Can you work these out from the model? Positions are in its coordinate system, mm. A direction names the side the tool comes from. Give positions to 0.01 mm unless a question says otherwise; leave off trailing zeros. Order: outer loops, then holes, each group sorted by start corner. A loop starts at its lowest first (then second) coordinate and runs counter-clockwise, first axis right, second up. Notation, with made-up numbers: (80.5, 46) - (94.5, 46) arc R22 cw to (94.5, 81) - close; hole circle Ø7 at (-21.5, 47). An arc over 180 degrees is marked (long way). Answer as CSV lines item,"result".
```python
from build123d import *

# Parameters (mm, degrees)
SKETCH1_R           = 200
BOSS_EXTRUDE1_DEPTH = 10
SKETCH2_R           = 6.25
CUT_EXTRUDE1_DEPTH  = 284.019433962
SKETCH4_R           = 2.55
CUT_EXTRUDE2_DEPTH  = 284.019433962
CIRPATTERN1_COUNT   = 8
SKETCH5_R           = 2.05
CUT_EXTRUDE3_DEPTH  = 284.019433962
CIRPATTERN2_COUNT   = 4
CUT_EXTRUDE4_START  = -10
CUT_EXTRUDE4_DEPTH  = 10
CIRPATTERN3_COUNT   = 4
SKETCH7_R           = 40
CUT_EXTRUDE5_DEPTH  = 282.602556807
FILLET1_R           = 10


with BuildPart() as part:
    # Sketch1 → Boss-Extrude1 (new body)
    with BuildSketch(Plane(origin=(0, 0, 0), x_dir=(1, 0, 0), z_dir=(0, 1, 0))):
        with Locations(Location((0, 0, 0), (0, 0, 270))):
            Circle(SKETCH1_R)
    extrude(amount=BOSS_EXTRUDE1_DEPTH)

    # Sketch2 → Cut-Extrude1 (cut, through all)
    with BuildSketch(Plane(origin=(0, 10, 0), x_dir=(1, 0, 0), z_dir=(0, 1, 0))):
        with Locations(Location((-135.764501988, 0, 0), (0, 0, 270))):
            Circle(SKETCH2_R)
        with Locations(Location((0, -135.764501988, 0), (0, 0, 270))):
            Circle(SKETCH2_R)
        with Locations(Location((135.764501988, 0, 0), (0, 0, 270))):
            Circle(SKETCH2_R)
        with Locations(Location((0, 135.764501988, 0), (0, 0, 270))):
            Circle(SKETCH2_R)
    extrude(amount=-CUT_EXTRUDE1_DEPTH, mode=Mode.SUBTRACT)

    # Sketch4 → Cut-Extrude2 (cut, through all)
    with BuildSketch(Plane(origin=(0, 10, 0), x_dir=(1, 0, 0), z_dir=(0, 1, 0))):
        with Locations(Location((20.090880199, 48.503675457, 0), (0, 0, 270))):
            Circle(SKETCH4_R)
    cut_extrude2 = extrude(amount=-CUT_EXTRUDE2_DEPTH, mode=Mode.SUBTRACT)

    # CirPattern1: Cut-Extrude2 ×8 about axis
    cirpattern1_axis = Axis((0, 0, 0), (0, 1, 0))
    for i in range(1, CIRPATTERN1_COUNT):
        add(cut_extrude2.rotate(cirpattern1_axis, i * 360 / CIRPATTERN1_COUNT), mode=Mode.SUBTRACT)

    # Sketch5 → Cut-Extrude3 (cut, through all)
    with BuildSketch(Plane(origin=(0, 10, 0), x_dir=(1, 0, 0), z_dir=(0, 1, 0))):
        with Locations(Location((-188.264501988, 8.25, 0), (0, 0, 270))):
            Circle(SKETCH5_R)
        with Locations(Location((-174.764501988, 8.25, 0), (0, 0, 270))):
            Circle(SKETCH5_R)
        with Locations(Location((-174.764501988, -8.25, 0), (0, 0, 270))):
            Circle(SKETCH5_R)
        with Locations(Location((-188.264501988, -8.25, 0), (0, 0, 270))):
            Circle(SKETCH5_R)
    cut_extrude3 = extrude(amount=-CUT_EXTRUDE3_DEPTH, mode=Mode.SUBTRACT)

    # CirPattern2: Cut-Extrude3 ×4 about axis
    cirpattern2_axis = Axis((0, 0, 0), (0, 1, 0))
    for i in range(1, CIRPATTERN2_COUNT):
        add(cut_extrude3.rotate(cirpattern2_axis, i * 360 / CIRPATTERN2_COUNT), mode=Mode.SUBTRACT)

    # Sketch6 → Cut-Extrude4 (cut)
    with BuildSketch(Plane(origin=(0, 10, 0), x_dir=(1, 0, 0), z_dir=(0, 1, 0)).offset(CUT_EXTRUDE4_START)):
        with BuildLine():
            Line((-198.997487421, 20), (-118.321595662, 20))
            ThreePointArc((-118.321595662, 20), (-84.852813742, 84.852813742), (-20, 118.321595662))
            Line((-20, 118.321595662), (-20, 198.997487421))
            ThreePointArc((-20, 198.997487421), (-141.421356237, 141.421356237), (-198.997487421, 20))
        make_face()
        with BuildLine():
            Line((-198.997487421, -20), (-198.997487421, 20))
            ThreePointArc((-198.997487421, 20), (-200, 0), (-198.997487421, -20))
        make_face()
    cut_extrude4 = extrude(amount=CUT_EXTRUDE4_DEPTH, mode=Mode.SUBTRACT)

    # CirPattern3: Cut-Extrude4 ×4 about axis
    cirpattern3_axis = Axis((0, 0, 0), (0, 1, 0))
    for i in range(1, CIRPATTERN3_COUNT):
        add(cut_extrude4.rotate(cirpattern3_axis, i * 360 / CIRPATTERN3_COUNT), mode=Mode.SUBTRACT)

    # Sketch7 → Cut-Extrude5 (cut, through all)
    with BuildSketch(Plane(origin=(0, 10, 0), x_dir=(1, 0, 0), z_dir=(0, 1, 0))):
        with Locations(Location((0, 0, 0), (0, 0, 270))):
            Circle(SKETCH7_R)
    extrude(amount=-CUT_EXTRUDE5_DEPTH, mode=Mode.SUBTRACT)

    # Fillet1
    fillet1_edges = [part.edges().sort_by_distance(p)[0] for p in [
        (-198.997487421, 5, -20),
        (-20, 5, -198.997487421),
        (-198.997487421, 5, 20),
        (-20, 5, 198.997487421),
        (198.997487421, 5, 20),
        (20, 5, -198.997487421),
        (20, 5, 198.997487421),
        (198.997487421, 5, -20),
    ]]
    fillet(fillet1_edges, radius=FILLET1_R)


solid = part.part
```
1) I want a section at A-A on z = 0. Write out the boundary of the cut face in (x, y).
Answer block:
outline,"(-199, 0) - (-142.01, 0) - (-142.01, 10) - (-199, 10) - close; (-129.51, 0) - (-40, 0) - (-40, 10) - (-129.51, 10) - close; (40, 0) - (129.51, 0) - (129.51, 10) - (40, 10) - close; (142.01, 0) - (199, 0) - (199, 10) - (142.01, 10) - close"
2) Which directions (+Z, -Z, +X, -X, +Y, -Y) give clear straight access to the entire face, cutting with the end or side of a thin tool? Please do faces 5 (the cylindrical face through (-196.15, 5.07, -16.99)), 6 (the flat face through (20, 5, 153)), 7 (the flat face through (20, 5, -154)), 8 (the flat face through (198.997, 5, 0)), 9 (the flat face through (-20, 5, 154)).
Answer block:
face 5,"-Z, -X, +Y, -Y"
face 6,"+Z, +X, +Y, -Y"
face 7,"-Z, +X, +Y, -Y"
face 8,"+Z, -Z, +X, +Y, -Y"
face 9,"+Z, -X, +Y, -Y"
3) I'm going to push flat-ended pins straight in: P1, Ø5, axis at y = 5, z = 137.5, coming from the +X side; P2, Ø4, axis at y = 5.5, z = -107, coming from the -X side; P3, Ø3, axis at x = -122, y = 1.5, coming from the -Z side. Where does each tip first touch, or does it pass through?
Answer block:
P1,"x = 20"
P2,"x = -58.09"
P3,"z = -20"
4) I want a section at C-C on z = -154.5. Write out the boundary of the cut face in (x, y).
Answer block:
outline,"(-20, 0) - (20, 0) - (20, 10) - (-20, 10) - close"
5) I want a section at D-D on y = 5.25. Count the separate pieces of the cut face and the enclosed holes in it, plus the area to 3 significant figures.
Answer block:
separate pieces,"1"
enclosed holes,"29"
area,"51,900 mm2"
6) I need wall thicknesses on line 1 along Z through (x, y) = (0.5, 6.25); line 2 along Z through (x, y) = (8.25, 6.75); line 3 along Z through (x, y) = (-8, 3.5). Which ranges of each line are inside material? Lowest first, please. Write a range as [from, to].
Answer block:
line 1,"[-199, -141.99], [-129.53, -40], [40, 129.53], [141.99, 199]"
line 2,"[-199, -190.31], [-186.21, -176.81], [-172.71, -39.14], [39.14, 172.71], [176.81, 186.21], [190.31, 199]"
line 3,"[-199, -190.3], [-186.23, -176.8], [-172.73, -39.19], [39.19, 172.73], [176.8, 186.23], [190.3, 199]"
7) If we mould it in two halves opening along X, with no side actions, what happens to faces 1 (the cylindrical face through (85.6, 4.9, 84.1)), 2 (the flat face through (-153, 5, 20)), 3 (the flat face through (-20, 5, -153)), 4 (the cylindrical face through (141.96, 5.07, -0.81))? For each: +X half, -X half, draft (parallel to the pull), parting line (faces both ways), or undercut.
Answer block:
face 1,"+X half"
face 2,"draft"
face 3,"-X half"
face 4,"undercut"
8) I want a section at B-B on x = 87. Write out the boundary of the cut face in (y, z).
Answer block:
outline,"(0, -82.65) - (10, -82.65) - (10, 82.65) - (0, 82.65) - close"
